For this review, take the finished solid that the model builds, in its own axes (mm). A direction names the side the tool comes from. Give positions to 0.01 mm unless a question says otherwise; leave off trailing zeros. Write each loop counter-clockwise with the first axis right and the second up, starting at its lowest first coordinate (ties: lowest second). Pieces come first, ordered by that corner, then holes.
1) Machinability: for faces 4 (the face through (1.65, 3.98, 0.01)), 5 (the face through (-9.74, -1.98, 0.01)), 6 (the face through (6.736, 3.638, 0.014)), which of the approach directions +Z, -Z, +X, -X, +Y, -Y give a long, thin tool a straight path to every point of the face, cutting with its end or side? Answer none if there is none.
2) Draft analysis for pull direction X (two halves, no side actions). For faces 1 (the face through (-8.772, 3.463, 0.014)), 2 (the face through (-3.1, 1.5, -1)), 3 (the face through (7.2, 0, 0)), state which applies: pulls with the +X half, pulls with the -X half, needs draft (parallel to the pull), parting line crosses it, or undercut.
3) We need section B-B on z = -0.5. Give the boundary of the cut face in (x, y), and give its area (3 significant figures).
4) Wall thickness on line 1 along Y through (x, z) = (-4, -0.35); line 2 along Y through (x, z) = (-16.75, -0.8); line 3 along Y through (x, z) = (4.2, -0.25): over which ranges is each line inside the solid? List them lowest first.
5) We need section C-C on y = -3. Give the boundary of the cut face in (x, z).
6) We need section D-D on x = 4.2. Give the boundary of the cut face in (y, z), and give its area (3 significant figures).
7) We need section A-A on x = -7.25. Give the boundary of the cut face in (y, z) (3 decimals), and give its area (3 significant figures).
from build123d import *

# Parameters (mm, degrees)
F1_DEPTH     = 1
F2_T1_DEPTH  = 2
F2_T3_DEPTH  = 4.1120925968
F2_T5_DEPTH  = 5.1335042229
F2_T7_DEPTH  = 4.211585233
F2_T9_DEPTH  = 4.4058060179
F2_T11_DEPTH = 4.5


# Not quite as in the source:
# - a fillet or chamfer that OpenCascade refuses, or shapes differently, is made with other operations: its cross-section is extruded or revolved along the edge and cut away or added


with BuildPart() as f1:
    # F0 (on Top) → F1 (new body, symmetric)
    with BuildSketch(Plane.XY):
        with BuildLine():
            Line((-19.8, -3.608959583), (-19.6536349592, -4.8))
            Line((-19.6536349592, -4.8), (7.2, -1.5))
            Line((7.2, -1.5), (7.2, 1.5))
            Line((7.2, 1.5), (5.5036997956, 1.7084556032))
            ThreePointArc((5.5036997956, 1.7084556032), (6.7140946083, 3.4735867022), (6.15341333, 5.5391084047))
            Line((6.15341333, 5.5391084047), (5.0809511096, 4.6392057511))
            ThreePointArc((5.0809511096, 4.6392057511), (4.2, 2.75), (3.3190488904, 4.6392057511))
            Line((3.3190488904, 4.6392057511), (2.24658667, 5.5391084047))
            ThreePointArc((2.24658667, 5.5391084047), (1.6526664248, 3.7834167399), (2.4044726286, 2.089314644))
            Line((2.4044726286, 2.089314644), (-19.6536349592, 4.8))
            Line((-19.6536349592, 4.8), (-19.8, 3.608959583))
            Line((-19.8, 3.608959583), (0, 0.4))
            Line((0, 0.4), (0, -0.4))
            Line((0, -0.4), (-19.8, -3.608959583))
        make_face()
    extrude(amount=F1_DEPTH, both=True)

    # F2: fillet of radius 0.5 on 14 edges, made by hand

    # F2_s2 → F2_t1 (join)
    with BuildSketch(Plane.XY.offset(-1)):
        with BuildLine():
            ThreePointArc((-0.4200093847, -0.4680703606), (-0.1192144254, -0.2985509875), (0, 0.0254896676))
            Line((0, 0.0254896676), (0, -0.4))
            Line((0, -0.4), (-0.4200093847, -0.4680703606))
        make_face()
        with BuildLine():
            ThreePointArc((0, -0.0254896676), (-0.1192144254, 0.2985509875), (-0.4200093847, 0.4680703606))
            Line((-0.4200093847, 0.4680703606), (0, 0.4))
            Line((0, 0.4), (0, -0.0254896676))
        make_face()
        with BuildLine():
            ThreePointArc((6.2414791759, 2.3719742233), (6.1818236662, 1.8762743647), (6.5807837768, 1.5760944855))
            Line((6.5807837768, 1.5760944855), (5.5036997956, 1.7084556032))
            ThreePointArc((5.5036997956, 1.7084556032), (5.9051744273, 2.003983077), (6.2414791759, 2.3719742233))
        make_face()
        with BuildLine():
            ThreePointArc((1.3273886474, 2.2216757617), (1.7871578534, 2.4163277766), (1.8492963629, 2.9117225034))
            ThreePointArc((1.8492963629, 2.9117225034), (2.0864966132, 2.4732542504), (2.4044726286, 2.089314644))
            Line((2.4044726286, 2.089314644), (1.3273886474, 2.2216757617))
        make_face()
    extrude(amount=F2_T1_DEPTH)

    # F2_s4 → F2_t3 (cut)
    with BuildSketch(Plane.XY.offset(-2.0560462984)):
        with BuildLine():
            ThreePointArc((3.1364686576, 4.3374940957), (3.1595895158, 4.6471438712), (2.995457531, 4.9107311415))
            Line((2.995457531, 4.9107311415), (3.3190488904, 4.6392057511))
            ThreePointArc((3.3190488904, 4.6392057511), (3.2161247629, 4.4953902231), (3.1364686576, 4.3374940957))
        make_face()
        with BuildLine():
            ThreePointArc((5.404542469, 4.9107311415), (5.2404104842, 4.6471438712), (5.2635313424, 4.3374940957))
            ThreePointArc((5.2635313424, 4.3374940957), (5.1838752371, 4.4953902231), (5.0809511096, 4.6392057511))
            Line((5.0809511096, 4.6392057511), (5.404542469, 4.9107311415))
        make_face()
    extrude(amount=F2_T3_DEPTH, mode=Mode.SUBTRACT)

    # F2_s6 → F2_t5 (cut)
    with BuildSketch(Plane.XY.offset(-2.5667521115)):
        with BuildLine():
            ThreePointArc((1.9057976578, 5.0131646836), (2.2511861931, 5.283864521), (2.6770350591, 5.1779193202))
            Line((2.6770350591, 5.1779193202), (2.24658667, 5.5391084047))
            ThreePointArc((2.24658667, 5.5391084047), (2.0599733824, 5.2866456202), (1.9057976578, 5.0131646836))
        make_face()
        with BuildLine():
            ThreePointArc((6.4942023422, 5.0131646836), (6.1488138069, 5.283864521), (5.7229649409, 5.1779193202))
            Line((5.7229649409, 5.1779193202), (6.15341333, 5.5391084047))
            ThreePointArc((6.15341333, 5.5391084047), (6.3400266176, 5.2866456202), (6.4942023422, 5.0131646836))
        make_face()
    extrude(amount=F2_T5_DEPTH, mode=Mode.SUBTRACT)

    # F2_s8 → F2_t7 (cut)
    with BuildSketch(Plane.XY.offset(-2.1057926165)):
        with BuildLine():
            ThreePointArc((7.2, 1.0576829534), (7.0744948043, 1.388973825), (6.7609854337, 1.5539497938))
            Line((6.7609854337, 1.5539497938), (7.2, 1.5))
            Line((7.2, 1.5), (7.2, 1.0576829534))
        make_face()
        with BuildLine():
            ThreePointArc((6.7609854337, -1.5539497938), (7.0744948043, -1.388973825), (7.2, -1.0576829534))
            Line((7.2, -1.0576829534), (7.2, -1.5))
            Line((7.2, -1.5), (6.7609854337, -1.5539497938))
        make_face()
    extrude(amount=F2_T7_DEPTH, mode=Mode.SUBTRACT)

    # F2_s10 → F2_t9 (cut)
    with BuildSketch(Plane.XY.offset(-2.202903009)):
        with BuildLine():
            ThreePointArc((-19.3250361256, -3.5319828216), (-19.644918404, -3.7253734495), (-19.7413123507, -4.0865282835))
            Line((-19.7413123507, -4.0865282835), (-19.8, -3.608959583))
            Line((-19.8, -3.608959583), (-19.3250361256, -3.5319828216))
        make_face()
        with BuildLine():
            ThreePointArc((-19.7413123507, 4.0865282835), (-19.644918404, 3.7253734495), (-19.3250361256, 3.5319828216))
            Line((-19.3250361256, 3.5319828216), (-19.8, 3.608959583))
            Line((-19.8, 3.608959583), (-19.7413123507, 4.0865282835))
        make_face()
    extrude(amount=F2_T9_DEPTH, mode=Mode.SUBTRACT)

    # F2_s12 → F2_t11 (cut)
    with BuildSketch(Plane.XY.offset(-2.25)):
        with BuildLine():
            ThreePointArc((-19.7146203929, -4.3037331596), (-19.5261439869, -4.6367845878), (-19.1573681188, -4.7390145663))
            Line((-19.1573681188, -4.7390145663), (-19.6536349592, -4.8))
            Line((-19.6536349592, -4.8), (-19.7146203929, -4.3037331596))
        make_face()
        with BuildLine():
            ThreePointArc((-19.1573681188, 4.7390145663), (-19.5261439869, 4.6367845878), (-19.7146203929, 4.3037331596))
            Line((-19.7146203929, 4.3037331596), (-19.6536349592, 4.8))
            Line((-19.6536349592, 4.8), (-19.1573681188, 4.7390145663))
        make_face()
    extrude(amount=F2_T11_DEPTH, mode=Mode.SUBTRACT)


solid = f1.part
Results list:
1. face 4: +Z, -Z
1. face 5: +Z, -Z, -X
1. face 6: +Z, -Z, +X
2. face 1: undercut
2. face 2: needs draft
2. face 3: pulls with the +X half
3. outline: (-19.74, -4.09) - (-19.71, -4.3) arc R0.5 ccw to (-19.16, -4.74) - (6.76, -1.55) arc R0.5 ccw to (7.2, -1.06) - (7.2, 1.06) arc R0.5 ccw to (6.76, 1.55) - (6.58, 1.58) arc R0.5 cw to (6.24, 2.37) arc R2.55 ccw to (6.49, 5.01) arc R0.5 ccw to (5.72, 5.18) - (5.4, 4.91) arc R0.5 ccw to (5.26, 4.34) arc R1.15 cw (long way) to (3.14, 4.34) arc R0.5 ccw to (3, 4.91) - (2.68, 5.18) arc R0.5 ccw to (1.91, 5.01) arc R2.55 ccw to (1.85, 2.91) arc R0.5 cw to (1.33, 2.22) - (-19.16, 4.74) arc R0.5 ccw to (-19.71, 4.3) - (-19.74, 4.09) arc R0.5 ccw to (-19.33, 3.53) - (-0.42, 0.47) arc R0.5 cw to (0, 0) arc R0.5 cw to (-0.42, -0.47) - (-19.33, -3.53) arc R0.5 ccw to start
3. area: 102 mm2
4. line 1: y = -2.88 to -1.05, 1.05 to 2.88
4. line 2: y = -4.44 to -3.11, 3.11 to 4.44
4. line 3: y = -1.87 to 2.75
5. outline: (-16.04, -1) - (-5.01, -1) - (-5.01, 1) - (-16.04, 1) - close
6. outline: (-1.87, -1) - (2.75, -1) - (2.75, 1) - (-1.87, 1) - close
6. area: 9.24 mm2
7. outline: (-3.276, -1) - (-1.575, -1) - (-1.575, 1) - (-3.276, 1) - close; (1.575, -1) - (3.276, -1) - (3.276, 1) - (1.575, 1) - close
7. area: 6.80 mm2
